Could you check a few things on this model? Use its own coordinates, in mm. Face numbers are marked on the shaded views. A direction names the side the tool comes from. Coordinates: 2 decimals unless noted, no trailing zeros. Write each loop counter-clockwise with the first axis right and the second up, starting at its lowest first coordinate (ties: lowest second). Pieces come first, ordered by that corner, then holes. Notation, with made-up numbers: M 24,59 L 42,59 A31 cw 42,93 Z; hole C 31,71.25 d6. An arc over 180 degrees is marked long. Answer as CSV lines item,"result". Start each with the question number.
Item 1: I'm going to push flat-ended pins straight in: P1, Ø2.5, axis at y = 2, z = 0, coming from the +X side; P2, Ø1.5, axis at y = 0.5, z = 1, coming from the -X side; P3, Ø3, axis at x = -2, z = -3, coming from the +Y side. Where does each tip first touch, or does it pass through?
Item 2: On a 3-axis mill with a long thin cutter (end or side, diameter ignored), from which of +Z, -Z, +X, -X, +Y, -Y can I reach the whole of each face in a straight line? I mean the marked faces 1, 2 and 3. Say none if no direction works.
Item 3: If I drill on line 1 along X through (y, z) = (-0.5, 0); line 2 along X through (y, z) = (-9, 1.5); line 3 along Z through (x, y) = (-11.75, -0.45), over which ranges is the centre line in solid material (lowest first)? Write a range as [from, to].
Item 4: Suppose I cut it at C-C, the plane y = -9.75. Write out the boundary of the cut face in (x, z).
Item 5: Suppose I cut it at B-B, the plane x = 11.75. Write out the boundary of the cut face in (y, z).
Item 6: Suppose I cut it at A-A, the plane x = 5.2. Write out the boundary of the cut face in (y, z), and give its area (3 significant figures).
Item 7: Suppose I cut it at D-D, the plane z = -3.5. Write out the boundary of the cut face in (x, y), and give its area (3 significant figures).
```python
from build123d import *

# Parameters (mm, degrees)
SKETCH1_W                = 19.6
SKETCH1_H                = 8.5
BOSS_EXTRUDE1_DEPTH      = 3.4
BOSS_EXTRUDE1_DEPTH_BACK = 17.25
SKETCH2_R                = 4.05
BOSS_EXTRUDE2_DEPTH      = 3.18
SKETCH4_W                = 3.95
SKETCH4_H                = 8.5
SKETCH4_R                = 0.75
BOSS_EXTRUDE3_DEPTH      = 0.7
FILLET1_R                = 4
SKETCH5_R                = 1.8
BOSS_EXTRUDE4_DEPTH      = 2.5
CHAMFER1_SIZE            = 2
CHAMFER1_SIZE2           = 2.856296013
CHAMFER1_PART_2_SIZE     = 2
CHAMFER1_PART_2_SIZE2    = 2.856296013


with BuildPart() as part:
    # Sketch1 → Boss-Extrude1 (new body, two sides)
    with BuildSketch(Plane(origin=(0, 0, 0), x_dir=(1, 0, 0), z_dir=(0, 1, 0))) as boss_extrude1_sk:
        Rectangle(SKETCH1_W, SKETCH1_H)
    extrude(amount=BOSS_EXTRUDE1_DEPTH)
    extrude(boss_extrude1_sk.sketch, amount=-BOSS_EXTRUDE1_DEPTH_BACK)

    # Sketch2 → Boss-Extrude2 (add)
    with BuildSketch(Plane(origin=(0, 3.4, 0), x_dir=(1, 0, 0), z_dir=(0, 1, 0))):
        with Locations((5.2, 0)):
            Circle(SKETCH2_R)
    extrude(amount=BOSS_EXTRUDE2_DEPTH)

    # Sketch4 → Boss-Extrude3 (add)
    with BuildSketch(Plane(origin=(0, 0, 0), x_dir=(1, 0, 0), z_dir=(0, 1, 0))):
        with Locations((11.775, 0)):
            Rectangle(SKETCH4_W, SKETCH4_H)
        with Locations((11.75, 0)):
            Circle(SKETCH4_R, mode=Mode.SUBTRACT)
        with Locations((-11.775, 0)):
            Rectangle(SKETCH4_W, SKETCH4_H)
        with Locations((-11.75, 0)):
            Circle(SKETCH4_R, mode=Mode.SUBTRACT)
    extrude(amount=-BOSS_EXTRUDE3_DEPTH)

    # Fillet1
    fillet1_edges = [part.edges().sort_by_distance(p)[0] for p in [
        (13.75, -0.35, -4.25),
        (13.75, -0.35, 4.25),
        (-13.75, -0.35, -4.25),
        (-13.75, -0.35, 4.25),
    ]]
    fillet(fillet1_edges, radius=FILLET1_R)

    # Sketch5 → Boss-Extrude4 (add)
    with BuildSketch(Plane(origin=(0, 6.58, 0), x_dir=(1, 0, 0), z_dir=(0, 1, 0))):
        with Locations((5.2, 0)):
            Circle(SKETCH5_R)
    extrude(amount=BOSS_EXTRUDE4_DEPTH)

    # Chamfer1
    chamfer1_edges = [part.edges().sort_by_distance(p)[0] for p in [
        (9.8, -17.25, 0),
    ]]
    chamfer1_side = [part.faces().sort_by_distance(p)[0] for p in [
        (9.8, -8.975, 0),
    ]]
    chamfer(chamfer1_edges, length=CHAMFER1_SIZE, length2=CHAMFER1_SIZE2, reference=chamfer1_side[0])

    # Chamfer1 part 2
    chamfer1_part_2_edges = [part.edges().sort_by_distance(p)[0] for p in [
        (-9.8, 3.4, 0),
    ]]
    chamfer1_part_2_side = [part.faces().sort_by_distance(p)[0] for p in [
        (-9.8, 1.7, 0),
    ]]
    chamfer(chamfer1_part_2_edges, length=CHAMFER1_PART_2_SIZE, length2=CHAMFER1_PART_2_SIZE2, reference=chamfer1_part_2_side[0])


solid = part.part
```
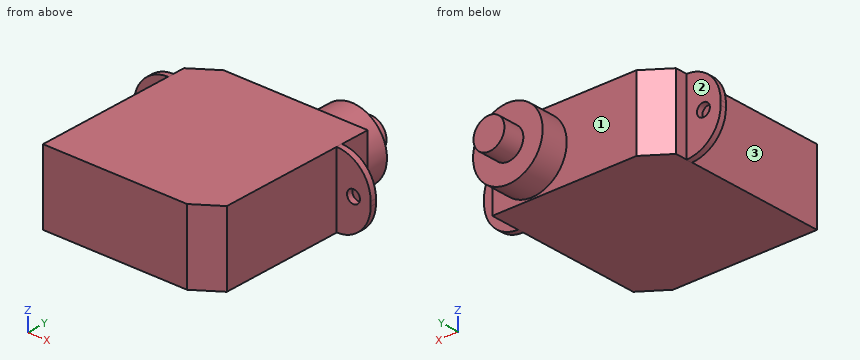
Ans:
1,P1,"stops at x = 9.8"
1,P2,"stops at x = -13.75"
1,P3,"stops at y = 3.4"
2,face 1,"+Y"
2,face 2,"+Z, -Z, -X, +Y"
2,face 3,"+Z, -Z, -X, -Y"
3,line 1,"x = [-13.75, -12.5], [-11, 11], [12.5, 13.75]"
3,line 2,"x = [-9.8, 9.8]"
3,line 3,"z = [-3.71, -0.75], [0.75, 3.71]"
4,outline,"M -9.8,-4.25 A4 ccw -9.75,-4.25 L 9.75,-4.25 A4 ccw 9.8,-4.25 L 9.8,4.25 A4 ccw 9.75,4.25 L -9.75,4.25 A4 ccw -9.8,4.25 Z"
5,outline,"M -0.7,-3.71 L 0,-3.71 L 0,-0.75 L -0.7,-0.75 Z; M -0.7,0.75 L 0,0.75 L 0,3.71 L -0.7,3.71 Z"
6,outline,"M -17.25,-4.25 L 3.4,-4.25 L 3.4,-4.05 L 6.58,-4.05 L 6.58,-1.8 L 9.08,-1.8 L 9.08,1.8 L 6.58,1.8 L 6.58,4.05 L 3.4,4.05 L 3.4,4.25 L -17.25,4.25 Z"
6,area,"210 mm^2"
7,outline,"M -12.08,-0.7 L -9.8,-0.7 L -9.8,-17.25 L 6.94,-17.25 L 9.8,-15.25 L 9.8,-0.7 L 12.08,-0.7 L 12.08,0 L 9.8,0 L 9.8,3.4 L 7.24,3.4 L 7.24,6.58 L 3.16,6.58 L 3.16,3.4 L -6.94,3.4 L -9.8,1.4 L -9.8,0 L -12.08,0 Z"
7,area,"415 mm^2"
